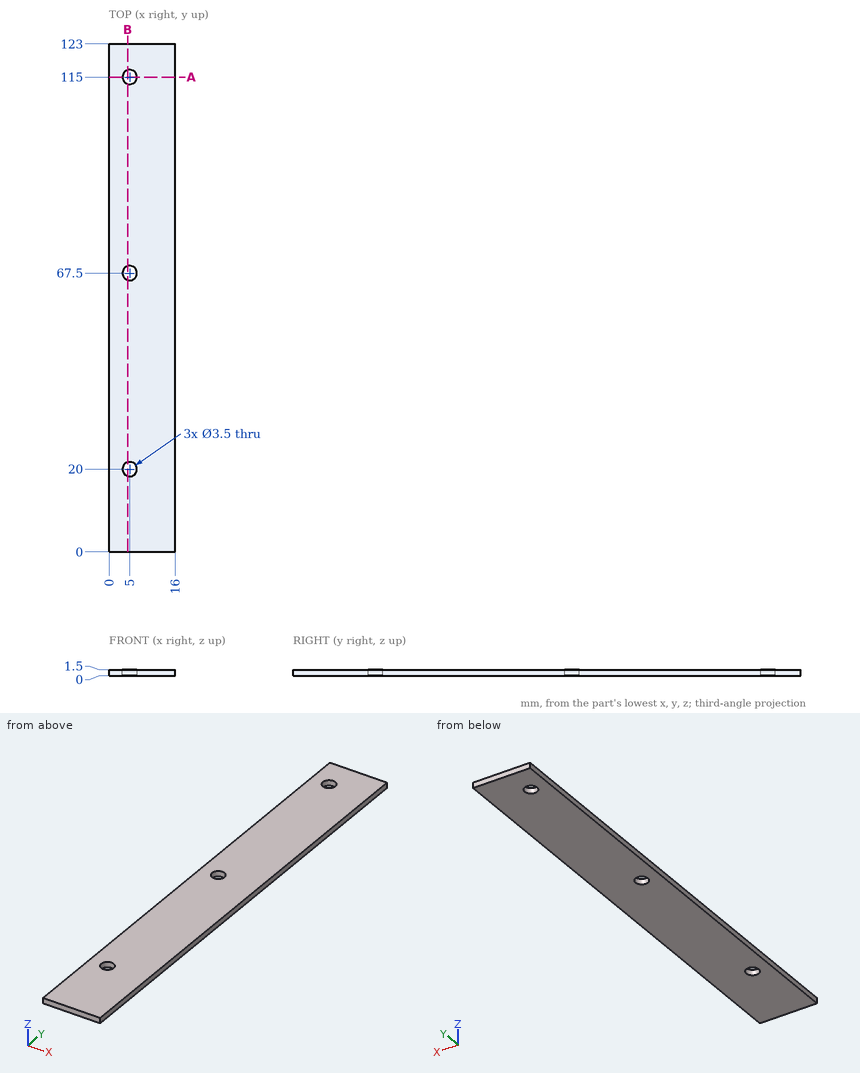
Check sheet for the drawn part. Datum: minimum x, y, z corner. Units: mm. Round coordinates to 2 decimals unless told otherwise and drop trailing zeros. Loops run counter-clockwise (first coordinate to the right, second up) from the corner with the lowest first, then second, coordinate; pieces in that order, holes last. Notation, with made-up numbers: (-30.75, -18.75) - (-7.75, -18.75) arc R25 ccw to (-7.75, -0.75) - close; hole circle Ø7 at (38, -7.5). An arc over 180 degrees is marked (long way). Use one line per item in the form item = value.
1. Gauge pin test, flat end, axial feed: pin 1 Ø4 at (x, y) = (5, 115) entering from -Z. Record the tip position at first contact, or that the pin passes through.
A:
pin_1 = 0
2. Scan lines: probe 1 along Y at (x, z) = (5, 0.4); probe 2 along X at (y, z) = (67.5, 0.8); probe 3 along Y at (x, z) = (6.5, 1.15). Record each from-to range of solid material in increasing order.
A:
probe_1 = 0 to 18.25, 21.75 to 65.75, 69.25 to 113.25, 116.75 to 123
probe_2 = 0 to 3.25, 6.75 to 16
probe_3 = 0 to 19.1, 20.9 to 66.6, 68.4 to 114.1, 115.9 to 123
3. Section check A-A on y = 115. Record the cut outline in (x, z), and give its area (4 significant figures).
A:
outline = (0, 0) - (3.25, 0) - (3.25, 1.5) - (0, 1.5) - close; (6.75, 0) - (16, 0) - (16, 1.5) - (6.75, 1.5) - close
area = 18.75 mm²
4. Section check B-B on x = 4.5. Record the cut outline in (y, z).
A:
outline = (0, 0) - (18.32, 0) - (18.32, 1.5) - (0, 1.5) - close; (21.68, 0) - (65.82, 0) - (65.82, 1.5) - (21.68, 1.5) - close; (69.18, 0) - (113.32, 0) - (113.32, 1.5) - (69.18, 1.5) - close; (116.68, 0) - (123, 0) - (123, 1.5) - (116.68, 1.5) - close
